For this review, take the finished solid that the model builds, in its own axes (mm). A direction names the side the tool comes from. Round coordinates to 2 decimals unless told otherwise and drop trailing zeros. Write each loop counter-clockwise with the first axis right and the second up, starting at its lowest first coordinate (ties: lowest second). Pieces come first, ordered by that corner, then holes. Notation, with made-up numbers: M -33,32 L -10,32 A28 ccw -10,64 Z; hole C -19,67.5 d4. An arc over 180 degrees is marked long. Use one line per item in the form item = value. Start each with the question number.
Item 1: Draft analysis for pull direction X (two halves, no side actions). For faces 1 (the flat face through (283.673, 166.408, 2.465)), 2 (the cylindrical face through (302.293, 234.883, 2.465)), 3 (the flat face through (347.51, 261.26, 2.46)), 4 (the cylindrical face through (313.49, 233.01, 2.46)), state which applies: released by +X, released by -X, zero draft, split by the parting line, or undercut.
Item 2: For line 1 (Y direction, x = 330, z = 4.55); line 2 (Y direction, x = 330.5, z = 3.65); line 3 (X direction, y = 196, z = 1.7), list the stretches that pass through material, from the lowest coordinate up. Write a range as [from, to].
Item 3: Add section B-B (x = 322.5). State the section outline as (y, z) points.
Item 4: For P1, Ø3, axis at x = 340.5, z = 2, coming from the +Y side; P2, Ø12, axis at x = 325.5, y = 203, coming from the -Z side; P3, Ø2.5, axis at y = 227.5, z = 1.5, coming from the -X side; P4, Ø1.5, axis at y = 259, z = 2.5, coming from the +X side, all flat-tipped, find the tip position at first contact; note any pin that passes through.
Item 5: Add section C-C (y = 177). State the section outline as (x, z) points, and give its area (3 significant figures).
Item 6: Add section A-A (z = 2.65). State the section outline as (x, y) points (3 decimals), and give its area (3 significant figures).
Item 7: For faces 5 (the flat face through (314.715, 210, 2)), 6 (the flat face through (280.18, 266.24, 2.46)), 7 (the cylindrical face through (351.77, 255.53, 2.46)), list the 3-axis set-ups (+Z, -Z, +X, -X, +Y, -Y) from which the entire face can be reached by the end or side of a thin tool; tool diameter is ignored.
from build123d import *

# Parameters (mm, degrees)
MODEL_R             = 3.25
BOSS_EXTRUDE1_DEPTH = 5


with BuildPart() as part:
    # Model → Boss-Extrude1 (new body)
    with BuildSketch(Plane.XY):
        with BuildLine():
            Line((350.531086943, 258.379089544), (344.410544625, 264.21942133))
            ThreePointArc((344.410544625, 264.21942133), (310.747790065, 279.802358255), (274.574415573, 271.586766634))
            Line((274.574415573, 271.586766634), (285.935808975, 260.74552029))
            ThreePointArc((285.935808975, 260.74552029), (308.96264008, 264.906909994), (330.701924732, 256.249218742))
            ThreePointArc((330.701924732, 256.249218742), (332.244741838, 253.385658556), (331.150021748, 250.322678066))
            Line((331.150021748, 250.322678066), (315.766337555, 234.200907326))
            ThreePointArc((315.766337555, 234.200907326), (313.453795395, 233.004786403), (310.89495725, 233.485310955))
            ThreePointArc((310.89495725, 233.485310955), (302.169602206, 234.857703267), (294.715316918, 230.11967497))
            Line((294.715316918, 230.11967497), (294.715316918, 222.972135785))
            ThreePointArc((294.715316918, 222.972135785), (294.657727687, 222.677637577), (294.643218038, 222.377912396))
            ThreePointArc((294.643218038, 222.377912396), (294.667183717, 221.884389879), (294.715316918, 221.392635851))
            Line((294.715316918, 221.392635851), (294.715316918, 208.14628496))
            ThreePointArc((294.715316918, 208.14628496), (294.681096364, 207.624180191), (294.579020223, 207.11100878))
            Line((294.579020223, 207.11100878), (272.456879039, 124.550053909))
            ThreePointArc((272.456879039, 124.550053909), (272.856480729, 121.514777728), (275.285306164, 119.651074423))
            Line((275.285306164, 119.651074423), (286.876416079, 116.545245882))
            ThreePointArc((286.876416079, 116.545245882), (289.91169226, 116.944847572), (291.775395565, 119.373673007))
            Line((291.775395565, 119.373673007), (314.579020223, 204.477958828))
            ThreePointArc((314.579020223, 204.477958828), (314.681096364, 204.991130239), (314.715316918, 205.513235008))
            Line((314.715316918, 205.513235008), (314.715316918, 215.05078415))
            Line((314.715316918, 215.05078415), (350.663575197, 252.723787))
            ThreePointArc((350.663575197, 252.723787), (351.768582577, 255.578877488), (350.531086943, 258.379089544))
        make_face()
        with Locations((304.715316918, 222.61967497)):
            Circle(MODEL_R, mode=Mode.SUBTRACT)
    extrude(amount=BOSS_EXTRUDE1_DEPTH)


solid = part.part
Calculated:
q1.face_1 = released by -X
q1.face_2 = undercut
q1.face_3 = released by +X
q1.face_4 = undercut
q2.line_1 = [231.07, 249.12], [256.78, 274.26]
q2.line_2 = [231.59, 249.64], [256.4, 274.01]
q2.line_3 = [291.6, 312.31]
q3.outline = M 223.21,0 L 241.26,0 L 241.26,5 L 223.21,5 Z; M 261.22,0 L 277.3,0 L 277.3,5 L 261.22,5 Z
q4.P1 = 268.78
q4.P2 = through
q4.P3 = 294.72
q4.P4 = 350.66
q5.outline = M 286.51,0 L 307.22,0 L 307.22,5 L 286.51,5 Z
q5.area = 104 mm^2
q6.outline = M 272.457,124.55 A4 ccw 275.285,119.651 L 286.876,116.545 A4 ccw 291.775,119.374 L 314.579,204.478 A4 ccw 314.715,205.513 L 314.715,215.051 L 350.664,252.724 A4 ccw 350.531,258.379 L 344.411,264.219 A57.5 ccw 274.574,271.587 L 285.936,260.746 A42.5 cw 330.702,256.249 A4 cw 331.15,250.323 L 315.766,234.201 A4 cw 310.895,233.485 A12.5 ccw 294.715,230.12 L 294.715,222.972 A2.075 ccw 294.643,222.378 A10.075 ccw 294.715,221.393 L 294.715,208.146 A4 cw 294.579,207.111 Z; hole C 304.715,222.62 d6.5
q6.area = 3,910 mm^2
q7.face_5 = +Z, -Z, +X, -Y
q7.face_6 = +Z, -Z, -X
q7.face_7 = +Z, -Z, +X
